Can you work these out from the model? Positions are in its coordinate system, mm. A direction names the side the tool comes from. Coordinates: 2 decimals unless noted, no trailing zeros. Loops run counter-clockwise (first coordinate to the right, second up) from the corner with the lowest first, then second, coordinate; pieces in that order, holes last.
```python
from build123d import *

# Parameters (mm, degrees)
F0_W     = 102
F0_H     = 102
F1_DEPTH = 3
F2_W     = 5
F2_H     = 3
F2_W_2   = 3.5
F3_DEPTH = 3
F4_W     = 3
F4_H     = 5
F5_DEPTH = 3


with BuildPart() as f1:
    # F0 (on Top) → F1 (new body)
    with BuildSketch(Plane.XY):
        Rectangle(F0_W, F0_H)
    extrude(amount=F1_DEPTH)

    # F2 (on face) → F3 (join, through all)
    with BuildSketch(Plane.XY.offset(3)):
        with Locations((0, 52.5)):
            Rectangle(F2_W, F2_H)
        with Locations((10, 52.5)):
            Rectangle(F2_W, F2_H)
        with Locations((20, 52.5)):
            Rectangle(F2_W, F2_H)
        with Locations((30, 52.5)):
            Rectangle(F2_W, F2_H)
        with Locations((40, 52.5)):
            Rectangle(F2_W, F2_H)
        with Locations((-10, 52.5)):
            Rectangle(F2_W, F2_H)
        with Locations((-30, 52.5)):
            Rectangle(F2_W, F2_H)
        with Locations((-40, 52.5)):
            Rectangle(F2_W, F2_H)
        with Locations((-20, 52.5)):
            Rectangle(F2_W, F2_H)
        with Locations((-10, -52.5)):
            Rectangle(F2_W, F2_H)
        with Locations((0, -52.5)):
            Rectangle(F2_W, F2_H)
        with Locations((10, -52.5)):
            Rectangle(F2_W, F2_H)
        with Locations((40, -52.5)):
            Rectangle(F2_W, F2_H)
        with Locations((-20, -52.5)):
            Rectangle(F2_W, F2_H)
        with Locations((-30, -52.5)):
            Rectangle(F2_W, F2_H)
        with Locations((-40, -52.5)):
            Rectangle(F2_W, F2_H)
        with Locations((20, -52.5)):
            Rectangle(F2_W, F2_H)
        with Locations((30, -52.5)):
            Rectangle(F2_W, F2_H)
        with Locations((-49.25, 52.5)):
            Rectangle(F2_W_2, F2_H)
        with Locations((49.25, 52.5)):
            Rectangle(F2_W_2, F2_H)
        with Locations((49.25, -52.5)):
            Rectangle(F2_W_2, F2_H)
        with Locations((-49.25, -52.5)):
            Rectangle(F2_W_2, F2_H)
    extrude(amount=-F3_DEPTH)

    # F4 (on face) → F5 (join)
    with BuildSketch(Plane.XY.offset(3)):
        with Locations((52.5, -5)):
            Rectangle(F4_W, F4_H)
        with Locations((52.5, -15)):
            Rectangle(F4_W, F4_H)
        with Locations((52.5, -25)):
            Rectangle(F4_W, F4_H)
        with Locations((52.5, -35)):
            Rectangle(F4_W, F4_H)
        with Locations((52.5, -45)):
            Rectangle(F4_W, F4_H)
        with Locations((52.5, 15)):
            Rectangle(F4_W, F4_H)
        with Locations((52.5, 45)):
            Rectangle(F4_W, F4_H)
        with Locations((52.5, 25)):
            Rectangle(F4_W, F4_H)
        with Locations((52.5, 5)):
            Rectangle(F4_W, F4_H)
        with Locations((52.5, 35)):
            Rectangle(F4_W, F4_H)
        with Locations((-52.5, -15)):
            Rectangle(F4_W, F4_H)
        with Locations((-52.5, -5)):
            Rectangle(F4_W, F4_H)
        with Locations((-52.5, 15)):
            Rectangle(F4_W, F4_H)
        with Locations((-52.5, 35)):
            Rectangle(F4_W, F4_H)
        with Locations((-52.5, -25)):
            Rectangle(F4_W, F4_H)
        with Locations((-52.5, 25)):
            Rectangle(F4_W, F4_H)
        with Locations((-52.5, -35)):
            Rectangle(F4_W, F4_H)
        with Locations((-52.5, 45)):
            Rectangle(F4_W, F4_H)
        with Locations((-52.5, -45)):
            Rectangle(F4_W, F4_H)
        with Locations((-52.5, 5)):
            Rectangle(F4_W, F4_H)
    extrude(amount=-F5_DEPTH)


solid = f1.part
```
(1) If I drill on probe 1 along X at (y, z) = (-42, 0.65), over which ranges is the centre line in solid material (lowest first)?
Check values:
probe 1: x = -51 to 51
(2) I want a section at A-A on x = 44. Write out the boundary of the cut face in (y, z).
Check values:
outline: (-51, 0) - (51, 0) - (51, 3) - (-51, 3) - close
(3) Which directions (+Z, -Z, +X, -X, +Y, -Y) give clear straight access to the entire face, cutting with the end or side of a thin tool? Please do faces 4 (the flat face through (37.5, 52, 2)), 5 (the flat face through (-53, 17.5, 2)), 6 (the flat face through (17.5, -53, 2)), 7 (the flat face through (52, 7.5, 2)).
Check values:
face 4: +Z, -Z, +Y
face 5: +Z, -Z, -X
face 6: +Z, -Z, -Y
face 7: +Z, -Z, +X
(4) I'm going to push flat-ended pins straight in: pin 1 (0.9 mm diameter, centred on x = 52.5, z = 1, fed in from -Y); pin 2 (0.9 mm diameter, centred on y = -52, z = 1.5, fed in from +X); pin 3 (0.9 mm diameter, centred on x = 14.5, z = 1, fed in from -Y). Where does each tip first touch, or does it pass through?
Check values:
pin 1: stops at y = -47.5
pin 2: stops at x = 51
pin 3: stops at y = -51
(5) If we mould it in two halves opening along X, with no side actions, what happens to faces 1 (the flat face through (54, -15, 2)), 2 (the flat face through (45, -51, 1)), 3 (the flat face through (-10, 54, 2))? For each: released by +X, released by -X, zero draft, split by the parting line, or undercut.
Check values:
face 1: released by +X
face 2: undercut
face 3: zero draft
